Can you work these out from the drawing? Everything is in mm from the part's minimum corner. A direction names the side the tool comes from. Round coordinates to 2 decimals unless told otherwise and drop trailing zeros. Write each loop counter-clockwise with the first axis right and the second up, starting at its lowest first coordinate (ties: lowest second). Pieces come first, ordered by that corner, then holes. Notation, with made-up numbers: (21.5, 55) - (80.5, 55) arc R14 ccw to (80.5, 78) - close; hole circle Ø3 at (-8, 88.25). An arc over 180 degrees is marked (long way). One line per item, written item: value. Start each with the question number.
(1) I want a section at D-D on x = 21. List the corners of the cut face in (y, z) for me (1 decimal).
(2) I want a section at A-A on z = 10.25. List the corners of the cut face in (x, y) for me (1 decimal).
(3) On a 3-axis mill with a long thin cutter (end or side, diameter ignored), from which of +Z, -Z, +X, -X, +Y, -Y can I reach the whole of each face in a straight line? I mean the marked faces 5, 6 and 7. Say none if no direction works.
(4) I want a section at C-C on z = 16.5. List the corners of the cut face in (x, y) for me (1 decimal).
(5) Thinking about a two-plate mould opening in X: for the marked faces 1, 2, 3 and 4, which applies, +X half, -X half, draft (parallel to the pull), parting line (faces both ways), or undercut?
(6) If I drill on L1, parallel to X at y = 7.5, z = 13; L2, parallel to Y at x = 8, z = 21.25; L3, parallel to X at y = 6.25, z = 15, over which ranges is the centre line in solid material (lowest first)? Write a range as from..to.
(7) I'm going to push flat-ended pins straight in: pin 1 Ø1.5 at (y, z) = (7, 11) entering from -X; pin 2 Ø2 at (y, z) = (8.5, 23) entering from -X; pin 3 Ø6 at (x, y) = (7.5, 2) entering from -Z (1 decimal); pin 4 Ø2.5 at (x, z) = (10.83, 21.5) entering from -Y. Where does each tip first touch, or does it pass through?
(8) I want a section at B-B on x = 10. Give the number of separate pieces and of enclosed holes in the cut face.
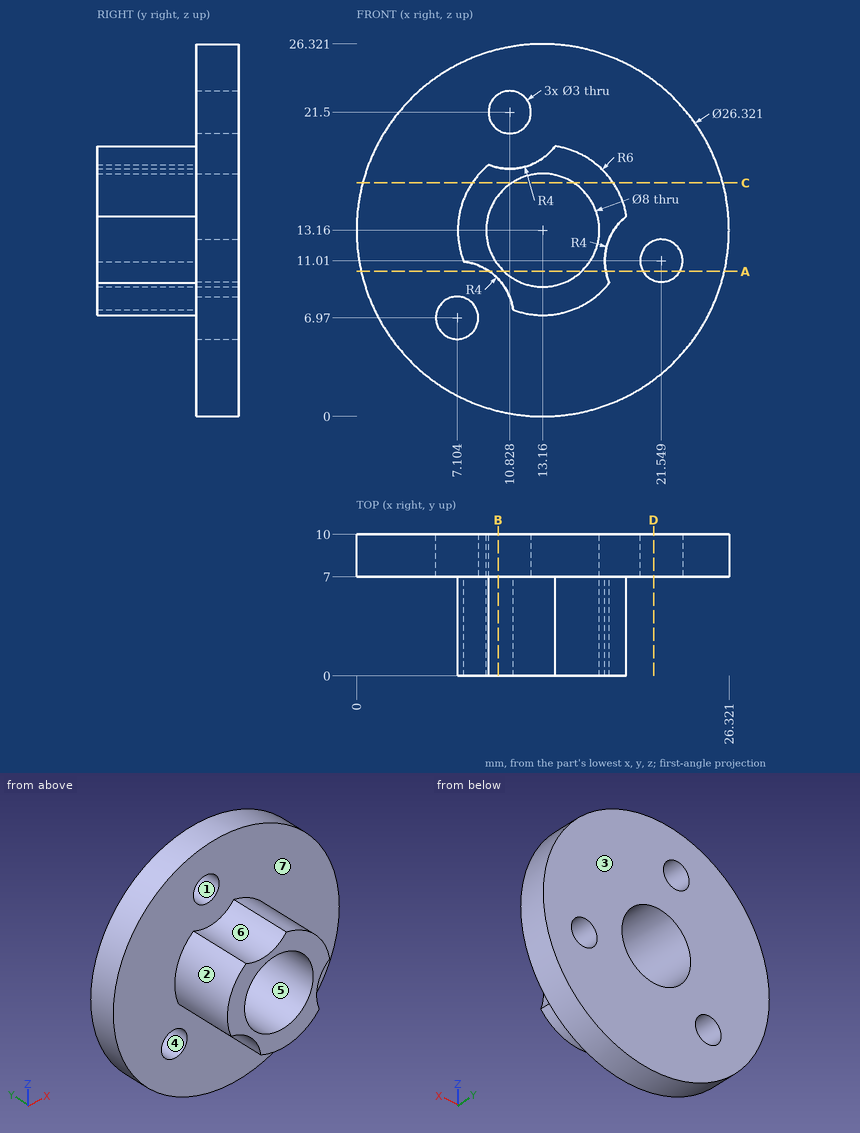
Established:
1. outline: (7, 2.6) - (10, 2.6) - (10, 9.6) - (7, 9.6) - close; (7, 12.4) - (10, 12.4) - (10, 23.7) - (7, 23.7) - close
2. outline: (0.3, 7) - (9.4, 7) - (9.4, 0) - (10.4, 0) - (10.4, 10) - (0.3, 10) - close; (15.9, 0) - (17.6, 0) - (17.6, 7) - (20.3, 7) - (20.3, 10) - (15.9, 10) - close; (22.8, 7) - (26, 7) - (26, 10) - (22.8, 10) - close
3. face 5: +Y, -Y
3. face 6: +Z, -Y
3. face 7: -Y
4. outline: (0.4, 7) - (8.2, 7) - (8.2, 0) - (11, 0) - (11, 10) - (0.4, 10) - close; (15.4, 0) - (18.1, 0) - (18.1, 7) - (25.9, 7) - (25.9, 10) - (15.4, 10) - close
5. face 1: undercut
5. face 2: -X half
5. face 3: draft
5. face 4: undercut
6. L1: 0..9.16, 17.16..26.32
6. L2: 7..10
6. L3: 7.45..9.61, 16.71..18.87
7. pin 1: x = 0.08
7. pin 2: x = 3.41
7. pin 3: z = 9.1
7. pin 4: through
8. separate pieces: 3
8. enclosed holes: 0
